Autodesk Inventor part; units mm, degrees
ref_plane "YZ Plane" through (0, 0, 0) normal (1, 0, 0) x (0, 1, 0)
ref_plane "XZ Plane" through (0, 0, 0) normal (0, 1, 0) x (-1, 0, 0)
ref_plane "XY Plane" through (0, 0, 0) normal (0, 0, 1) x (1, 0, 0)
sketch "Sketch1" plane through (0, 0, 0) normal (0, 0, 1) x (1, 0, 0)
  line L0 (0, 0) -> (430, 0)
  line L1 (430, 0) -> (430, 60)
  line L2 (430, 60) -> (0, 60)
  line L3 (0, 60) -> (0, 0)
  line L4 (215, 44.8722) -> (215, 13.4403) construction
  point P0 (27.5, 47.5)
  point P1 (402.5, 47.5)
  point P2 (0, 30)
  dimension "d0" = 430
  dimension "d1" = 60
  dimension "d4" = 375
  dimension "d9" = 215
  dimension "d10" = 12.5
extrude "Extrusion1" add sketch "Sketch1" along normal blind 3
hole "Hole1" at (27.5, 47.5, 0) at (402.5, 47.5, 0) direction (0, 0, 1) diameter 6.6 end through all
properties part number "light-trap-panel-bottom-front"
Here's how the part is built. I have some questions about the finished solid (model axes, mm). Coordinates: 2 decimals unless noted, no trailing zeros. Return JSON: item names as keys, results as strings. Group by question number.
Item 1: Will these pins go through, and if not, where does the flat tip stop? P1, Ø4, axis at x = 213, y = 33, coming from the -Z side; P2, Ø5.5, axis at x = 27.5, y = 47.5, coming from the -Z side.
Item 2: We'd pull the mould along X, two halves only. Please class faces 1 (the face through (212, 30, 0)), 2 (the face through (27.4, 44.2, 1.5)): +X half, -X half, draft (parallel to the pull), parting line (faces both ways), or undercut.
Item 3: I need wall thicknesses on line 1 (X direction, y = 47.5, z = 0.65); line 2 (Y direction, x = 27.5, z = 0.7); line 3 (X direction, y = 45.5, z = 1.3). Which ranges of each line are inside material? Lowest first, please. Write a range as from..to.
Calculated:
{
 "1": {"P1": "stops at z = 0", "P2": "passes through"},
 "2": {"face 1": "draft", "face 2": "undercut"},
 "3": {"line 1": "x = 0..24.2, 30.8..399.2, 405.8..430", "line 2": "y = 0..44.2, 50.8..60", "line 3": "x = 0..24.88, 30.12..399.88, 405.12..430"}
}
